```python
from build123d import *

# Parameters (mm, degrees)
F0_R     = 9.525
F0_R_2   = 6.35
F1_DEPTH = 6.35
F2_DEPTH = 3.175
F3_R     = 3.175


with BuildPart() as f1:
    # F0 (on Front) → F1 (new body)
    with BuildSketch(Plane.XZ):
        Circle(F0_R)
        Circle(F0_R_2, mode=Mode.SUBTRACT)
    extrude(amount=F1_DEPTH)

    # F0 (on Front) → F2 (join)
    with BuildSketch(Plane.XZ):
        Circle(F0_R_2)
    extrude(amount=F2_DEPTH)

    # F3
    f3_edges = [f1.edges().sort_by_distance(p)[0] for p in [
        (-9.525, 0, 0),
    ]]
    fillet(f3_edges, radius=F3_R)


solid = f1.part
```
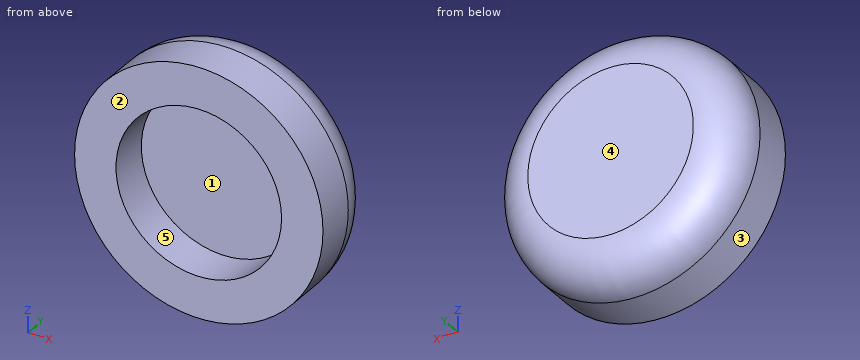
Check sheet for the modelled part. Datum: model origin and axes. Units: mm. Face numbers are marked on the shaded views. A direction names the side the tool comes from. Coordinates: 2 decimals unless noted, no trailing zeros. Order: outer loops, then holes, each group sorted by start corner. A loop starts at its lowest first (then second) coordinate and runs counter-clockwise, first axis right, second up. Notation, with made-up numbers: (36, 20) -> (72, 20) arc R14 cw to (72, 39) -> close; hole circle Ø3 at (10, 67.25). An arc over 180 degrees is marked (long way). Write item = value, one per line. Start each with the question number.
1) Cross-section at A-A (z = 0). Enter the section's corners in (x, y) (3 decimals).
2) Go/stop test with flat-tipped pins: P1, Ø1, axis at x = -4, z = -3, coming from the -Y side (3 decimals); P2, Ø2, axis at y = -3, z = -4, coming from the +X side; P3, Ø10, axis at x = -3, z = 0.5, coming from the -Y side; P4, Ø1.5, axis at x = -6, y = -5.5, coming from the +Z side. Record where each tip stops, or that it passes through.
3) Access from +Z, -Z, +X, -X, +Y, -Y to the whole of each face (thin tool, end or side, straight path). Record for the marked faces 4 and 5.
4) Cross-section at B-B (x = 0). Enter the section's corners in (y, z) (3 decimals).
5) Cross-section at C-C (y = -3.5). Enter the section's corners in (x, z) (3 decimals), then the cut area to 3 significant figures.
6) Cross-section at D-D (y = -0.5). Enter the section's corners in (x, z).
7) Material ranges on L1, parallel to Z at x = 0, y = -3.9 (3 decimals); L2, parallel to Y at x = -1, z = 4.5 (3 decimals); L3, parallel to Z at x = 4.5, y = -4.5, recorded low to high.
8) Mould release check, pull along X, two halves, no side actions. Record for the marked faces 1, 2 and 3: +X half, -X half, draft (parallel to the pull), parting line (faces both ways), or undercut.
Ans:
q1.outline = (-9.525, -6.35) -> (-6.35, -6.35) -> (-6.35, -3.175) -> (6.35, -3.175) -> (6.35, -6.35) -> (9.525, -6.35) -> (9.525, -3.175) arc R3.175 ccw to (6.35, 0) -> (-6.35, 0) arc R3.175 ccw to (-9.525, -3.175) -> close
q2.P1 = -3.175
q2.P2 = 9.04
q2.P3 = -6.35
q2.P4 = 7.95
q3.face_4 = +Z, -Z, +X, -X, +Y
q3.face_5 = -Y
q4.outline = (-6.35, -9.525) -> (-3.175, -9.525) arc R3.175 ccw to (0, -6.35) -> (0, 6.35) arc R3.175 ccw to (-3.175, 9.525) -> (-6.35, 9.525) -> (-6.35, 6.35) -> (-3.175, 6.35) -> (-3.175, -6.35) -> (-6.35, -6.35) -> close
q5.outline = circle Ø19.05 at (0, 0); hole circle Ø12.7 at (0, 0)
q5.area = 158 mm²
q6.outline = circle Ø16.12 at (0, 0)
q7.L1 = -9.525 to -6.35, 6.35 to 9.525
q7.L2 = -3.175 to 0
q7.L3 = -8.39 to -4.48, 4.48 to 8.39
q8.face_1 = undercut
q8.face_2 = draft
q8.face_3 = parting line
